Solid Edge part; units mm, degrees
sketch "Sketch1" plane through (0, 0, 0) normal (1, 0, 0) x (0, 1, 0)
  line L0 (-100, -3) -> (-100, -73)
  line L1 (-100, -73) -> (-97, -73)
  line L2 (-97, -73) -> (-97, -223)
  line L3 (-97, -223) -> (-100, -223)
  line L4 (-100, -223) -> (-100, -300)
  line L5 (-100, -300) -> (0, -300)
  line L6 (0, 0) -> (0, -300)
  line L7 (-50, 0) -> (0, 0)
  line L8 (-50, -3) -> (-50, 0)
  line L9 (-100, -3) -> (-50, -3)
  dimension "D1" = 50
  dimension "D2" = 50
  dimension "D3" = 97
  dimension "D4" = 100
extrude "Protrusion1" add sketch "Sketch1" along normal blind 3
mirror "Mirror1" about plane through (0, 0, 0) normal (0, -1, 0) of "Protrusion1"
sketch "Sketch2" plane through (3, 0, -150) normal (1, 0, 0) x (0, 1, 0)
  circle A0 centre (-50.4, -25.72) radius 1.25
  circle A1 centre (37.6, -25.72) radius 1.25
  circle A2 centre (37.6, -89.72) radius 1.25
  circle A3 centre (-50.4, -89.72) radius 1.25
  line L0 (-41.93, -137.43) -> (-41.93, -97.43)
  line L1 (-41.93, -97.43) -> (-44.93, -97.43)
  line L2 (-44.93, -97.43) -> (-44.93, -137.43)
  line L3 (-44.93, -137.43) -> (-41.93, -137.43)
  line L4 (-46.4, -31.72) -> (-46.4, -83.72)
  line L5 (-46.4, -83.72) -> (33.6, -83.72)
  line L6 (33.6, -83.72) -> (33.6, -31.72)
  line L7 (33.6, -31.72) -> (-46.4, -31.72)
  dimension "D1" = 33.6
  dimension "D2" = 33.6
  dimension "D3" = 50.4
  dimension "D4" = 41.93
  dimension "D5" = 44.93
  dimension "D6" = 41.93
extrude "Cutout1" cut sketch "Sketch2" against normal up to surface (3 mm away)
properties material "Acier"
Read the model definition and answer for the solid it produces. Units are mm, in the model's axes. Give positions to 0.01 mm unless a question says otherwise; leave off trailing zeros. Loops run counter-clockwise (first coordinate to the right, second up) from the corner with the lowest first, then second, coordinate; pieces in that order, holes last.
Item 1: Each of these flat-tipped pins is pushed along its axis until it touches: pin 1 Ø0.9 at (x, z) = (2, -201.5) entering from -Y; pin 2 Ø1.5 at (x, z) = (1, -158.5) entering from +Y; pin 3 Ø1.5 at (x, y) = (1.5, 80) entering from +Z. Where does it stop, or does it pass through?
Item 2: Find the intervals of material crossed by line 1 along Z through (x, y) = (1.85, 37.6); line 2 along Y through (x, z) = (0.6, -239.72); line 3 along Z through (x, y) = (1.6, -50.4), in increasing order.
Item 3: The part is cut by section B-B (y = 9.5). Write down the section's boundary in (x, z).
Item 4: The part is cut by section C-C (z = -107). Write down the section's boundary in (x, y).
Item 5: The part is cut by section A-A (x = 0.55). Write down the section's boundary in (y, z).
Taken from the geometry:
1. pin 1: stops at y = -97
1. pin 2: stops at y = 97
1. pin 3: stops at z = -3
2. line 1: z = -300 to -240.97, -238.47 to -176.97, -174.47 to 0
2. line 2: y = -100 to -51.65, -49.15 to 36.35, 38.85 to 100
2. line 3: z = -300 to -240.97, -238.47 to -176.97, -174.47 to -3
3. outline: (0, -300) - (3, -300) - (3, -233.72) - (0, -233.72) - close; (0, -181.72) - (3, -181.72) - (3, 0) - (0, 0) - close
4. outline: (0, -97) - (3, -97) - (3, 97) - (0, 97) - close
5. outline: (-100, -300) - (100, -300) - (100, -223) - (97, -223) - (97, -73) - (100, -73) - (100, -3) - (50, -3) - (50, 0) - (-50, 0) - (-50, -3) - (-100, -3) - (-100, -73) - (-97, -73) - (-97, -223) - (-100, -223) - close; hole circle Ø2.5 at (-50.4, -239.72); hole circle Ø2.5 at (-50.4, -175.72); hole (-46.4, -233.72) - (33.6, -233.72) - (33.6, -181.72) - (-46.4, -181.72) - close; hole (-44.93, -287.43) - (-41.93, -287.43) - (-41.93, -247.43) - (-44.93, -247.43) - close; hole circle Ø2.5 at (37.6, -239.72); hole circle Ø2.5 at (37.6, -175.72)
